Part model, mm, in its own coordinate system. A direction names the side the tool comes from. Give positions to 0.01 mm unless a question says otherwise; leave off trailing zeros. Write each loop counter-clockwise with the first axis right and the second up, starting at its lowest first coordinate (ties: lowest second). Pieces come first, ordered by that corner, then holes. Notation, with made-up numbers: M 57.5,-5.75 L 84.5,-5.75 A22 ccw 84.5,32.25 Z; hole C 44,26 d2. An arc over 180 degrees is marked long. Use a Markdown table: item, result.
```python
from build123d import *

# Parameters (mm, degrees)
BOSS_EXTRUDE1_DEPTH = 3
SKETCH2_R           = 1.5
SKETCH2_W           = 14
SKETCH2_H           = 12
CUT_EXTRUDE1_DEPTH  = 88.418533504
SKETCH3_R           = 1
SKETCH3_R_2         = 1.25
CUT_EXTRUDE2_DEPTH  = 88.418533504


with BuildPart() as part:
    # Sketch1 → Boss-Extrude1 (new body)
    with BuildSketch(Plane.XY):
        Polygon((0, 0), (22.5, 0), (22.5, -6), (47.5, -6), (47.5, 0), (70, 0), (70, 17.5), (73, 17.5), (73, 27.5), (70, 27.5), (70, 45), (47.5, 45), (47.5, 48), (22.5, 48), (22.5, 45), (0, 45), (0, 27.5), (-3, 27.5), (-3, 17.5), (0, 17.5), align=None)
    extrude(amount=BOSS_EXTRUDE1_DEPTH)

    # Sketch2 → Cut-Extrude1 (cut, through all)
    with BuildSketch(Plane.XY.offset(3)):
        with Locations((23, 10)):
            Circle(SKETCH2_R)
        with Locations((47, 10)):
            Circle(SKETCH2_R)
        with Locations((35, 6)):
            Rectangle(SKETCH2_W, SKETCH2_H)
    extrude(amount=-CUT_EXTRUDE1_DEPTH, mode=Mode.SUBTRACT)

    # Sketch3 → Cut-Extrude2 (cut, through all)
    with BuildSketch(Plane(origin=(0, 0, 0), x_dir=(-1, 0, 0), z_dir=(0, 0, -1))):
        with Locations((-51.881943016, 3)):
            Circle(SKETCH3_R)
        with Locations((-51.866980094, 7.122494405)):
            Circle(SKETCH3_R)
        with Locations((-50.860122949, 11.120171569)):
            Circle(SKETCH3_R)
        with Locations((-48.920581694, 14.757940628)):
            Circle(SKETCH3_R)
        with Locations((-46.162414669, 17.82187579)):
            Circle(SKETCH3_R)
        with Locations((-42.74782103, 20.131796631)):
            Circle(SKETCH3_R)
        with Locations((-38.877602325, 21.55186395)):
            Circle(SKETCH3_R)
        with Locations((-34.779353984, 21.998568038)):
            Circle(SKETCH3_R)
        with Locations((-30.694081142, 21.445639629)):
            Circle(SKETCH3_R)
        with Locations((-26.862025891, 19.925594708)):
            Circle(SKETCH3_R)
        with Locations((-23.508539385, 17.527822354)):
            Circle(SKETCH3_R)
        with Locations((-20.830829653, 14.39332804)):
            Circle(SKETCH3_R)
        with Locations((-18.98636441, 10.706441551)):
            Circle(SKETCH3_R)
        with Locations((-18.083610875, 6.683977124)):
            Circle(SKETCH3_R)
        with Locations((-18.175657153, 2.562483282)):
            Circle(SKETCH3_R)
        with Locations((-13.135450788, 2.562483282)):
            Circle(SKETCH3_R_2)
        with Locations((-13.046954317, 6.436588053)):
            Circle(SKETCH3_R_2)
        with Locations((-13.639570111, 10.266121435)):
            Circle(SKETCH3_R_2)
        with Locations((-14.894911752, 13.932268836)):
            Circle(SKETCH3_R_2)
        with Locations((-16.774031178, 17.321284856)):
            Circle(SKETCH3_R_2)
        with Locations((-19.21862708, 20.328022337)):
            Circle(SKETCH3_R_2)
        with Locations((-22.152853752, 22.859194643)):
            Circle(SKETCH3_R_2)
        with Locations((-25.485674269, 24.836269959)):
            Circle(SKETCH3_R_2)
        with Locations((-29.113684986, 26.197907811)):
            Circle(SKETCH3_R_2)
        with Locations((-32.924323727, 26.901862204)):
            Circle(SKETCH3_R_2)
        with Locations((-36.799362123, 26.926292344)):
            Circle(SKETCH3_R_2)
        with Locations((-40.61857375, 26.270440264)):
            Circle(SKETCH3_R_2)
        with Locations((-44.263464258, 24.954654343)):
            Circle(SKETCH3_R_2)
        with Locations((-47.62094776, 23.01975798)):
            Circle(SKETCH3_R_2)
        with Locations((-50.586855421, 20.52578301)):
            Circle(SKETCH3_R_2)
        with Locations((-53.069167386, 17.550107169)):
            Circle(SKETCH3_R_2)
        with Locations((-54.990867776, 14.185053378)):
            Circle(SKETCH3_R_2)
        with Locations((-56.29233417, 10.535025347)):
            Circle(SKETCH3_R_2)
        with Locations((-56.933187446, 6.713268358)):
            Circle(SKETCH3_R_2)
        with Locations((-56.893544575, 2.838355734)):
            Circle(SKETCH3_R_2)
    extrude(amount=-CUT_EXTRUDE2_DEPTH, mode=Mode.SUBTRACT)


solid = part.part
```
1. Cut at B-B, the plane y = 31. Give the cut face in (x, z).
Findings below:
| item | result |
|---|---|
| outline | M 0,0 L 70,0 L 70,3 L 0,3 Z |
2. Tool access for faces 1 (the flat face through (35, -6, 1)), 2 (the flat face through (47.5, -3, 1)), 3 (the flat face through (35, 0, 2)): list every direction of +Z, -Z, +X, -X, +Y, -Y with a clear straight run to the whole face (end or side of a thin tool).
Findings below:
| item | result |
|---|---|
| face 1 | +Z, -Z, +X, -X, -Y |
| face 2 | +Z, -Z, +X, -Y |
| face 3 | +Z, -Z |
3. Two-plate mould, pull along X, no slides. Class faces 4 (the flat face through (-1, 27.5, 1)), 5 (the flat face through (42, 6, 2)), 6 (the flat face through (73, 22, 1)): released by +X, released by -X, zero draft, split by the parting line, or undercut.
Findings below:
| item | result |
|---|---|
| face 4 | zero draft |
| face 5 | undercut |
| face 6 | released by +X |
4. Cut at C-C, the plane z = 2.4. State how many separate pieces and enclosed holes the cut face has, then the cut area to 3 significant figures.
Findings below:
| item | result |
|---|---|
| separate pieces | 1 |
| enclosed holes | 38 |
| area | 3,110 mm2 |
5. Drop flat-ended pins along their axis: P1, Ø1.5, axis at x = 8.5, z = 2, coming from the -Y side; P2, Ø1.2, axis at x = 23.51, y = 17.53, coming from the -Z side; P3, Ø0.9, axis at x = 10.5, z = 2, coming from the +Y side. Give the stop position or say it passes through.
Findings below:
| item | result |
|---|---|
| P1 | y = 0 |
| P2 | through |
| P3 | y = 45 |
6. Cut at A-A, the plane x = 60.5. Give the cut face in (y, z), then the cut area to 3 significant figures.
Findings below:
| item | result |
|---|---|
| outline | M 0,0 L 45,0 L 45,3 L 0,3 Z |
| area | 135 mm2 |
7. Drill centre lines: L1, parallel to X at y = 28, z = 1.85; L2, parallel to Y at x = 46, z = 1.6; L3, parallel to Y at x = 35.5, z = 1.6. Where is each one in solid material? Low to high.
Findings below:
| item | result |
|---|---|
| L1 | 0 to 32.33, 33.52 to 36.16, 37.44 to 70 |
| L2 | -6 to 8.88, 11.12 to 16.84, 18.81 to 48 |
| L3 | -6 to 0, 12 to 21.31, 22.69 to 48 |
